```python
from build123d import *

# Parameters (mm, degrees)
ESQUISSE1_W             = 60
ESQUISSE1_H             = 42
BOSS_EXTRU_1_DEPTH      = 35.125
COQUE4_T                = -3
ESQUISSE7_W             = 54
ESQUISSE7_H             = 36
BOSS_EXTRU_2_DEPTH      = 10.125
ESQUISSE8_W             = 60
ESQUISSE8_H             = 35.125
ENL_V_MAT_EXTRU_1_DEPTH = 1
ESQUISSE9_W             = 10
ESQUISSE9_H             = 22
BOSS_EXTRU_3_DEPTH      = 1
ESQUISSE10_W            = 18
ESQUISSE10_H            = 10
ENL_V_MAT_EXTRU_2_DEPTH = 3
ESQUISSE13_W            = 42
ESQUISSE13_H            = 22
ENL_V_MAT_EXTRU_3_DEPTH = 10
ESQUISSE15_W            = 7.326333239
ESQUISSE15_H            = 18.950794871
ENL_V_MAT_EXTRU_4_DEPTH = 4
ESQUISSE16_W            = 5
ESQUISSE16_H            = 6
BOSS_EXTRU_4_DEPTH      = 3


with BuildPart() as part:
    # Esquisse1 → Boss.-Extru.1 (new body)
    with BuildSketch(Plane.XY):
        with Locations((30, 21)):
            Rectangle(ESQUISSE1_W, ESQUISSE1_H)
    extrude(amount=BOSS_EXTRU_1_DEPTH)

    # Coque4
    coque4_openings = [part.faces().sort_by_distance(p)[0] for p in [
        (30, 21, 35.125),
    ]]
    offset(amount=COQUE4_T, openings=coque4_openings, kind=Kind.INTERSECTION)

    # Esquisse7 → Boss.-Extru.2 (add)
    with BuildSketch(Plane.XY.offset(3)):
        with Locations((30, 21)):
            Rectangle(ESQUISSE7_W, ESQUISSE7_H)
    extrude(amount=BOSS_EXTRU_2_DEPTH)

    # Esquisse8 → Enlèv. mat.-Extru.1 (cut)
    with BuildSketch(Plane(origin=(0, 42, 0), x_dir=(1, 0, 0), z_dir=(0, 1, 0))):
        with Locations((30, -17.5625)):
            Rectangle(ESQUISSE8_W, ESQUISSE8_H)
    extrude(amount=-ENL_V_MAT_EXTRU_1_DEPTH, mode=Mode.SUBTRACT)

    # Esquisse9 → Boss.-Extru.3 (add)
    with BuildSketch(Plane(origin=(0, 41, 0), x_dir=(1, 0, 0), z_dir=(0, 1, 0))):
        with Locations((55, -24.125)):
            Rectangle(ESQUISSE9_W, ESQUISSE9_H)
    extrude(amount=-BOSS_EXTRU_3_DEPTH)

    # Esquisse10 → Enlèv. mat.-Extru.2 (cut)
    with BuildSketch(Plane.ZY):
        with Locations((22.395110195, 7.568318588)):
            Rectangle(ESQUISSE10_W, ESQUISSE10_H)
    extrude(amount=-ENL_V_MAT_EXTRU_2_DEPTH, mode=Mode.SUBTRACT)

    # Esquisse13 → Enlèv. mat.-Extru.3 (cut)
    with BuildSketch(Plane(origin=(0, 39, 0), x_dir=(-1, 0, 0), z_dir=(0, -1, 0))):
        with Locations((-24, -24.125)):
            Rectangle(ESQUISSE13_W, ESQUISSE13_H)
    extrude(amount=-ENL_V_MAT_EXTRU_3_DEPTH, mode=Mode.SUBTRACT)

    # Esquisse15 → Enlèv. mat.-Extru.4 (cut)
    with BuildSketch(Plane(origin=(0, 41, 0), x_dir=(1, 0, 0), z_dir=(0, 1, 0))):
        with Locations((48.66316662, -25.649602565)):
            Rectangle(ESQUISSE15_W, ESQUISSE15_H)
    extrude(amount=-ENL_V_MAT_EXTRU_4_DEPTH, mode=Mode.SUBTRACT)

    # Esquisse16 → Boss.-Extru.4 (add)
    with BuildSketch(Plane.XY.offset(13.125)):
        with Locations((5.5, 38)):
            Rectangle(ESQUISSE16_W, ESQUISSE16_H)
    extrude(amount=BOSS_EXTRU_4_DEPTH)


solid = part.part
```
For this review, take the finished solid that the model builds, in its own axes (mm). A direction names the side the tool comes from. Round coordinates to 2 decimals unless told otherwise and drop trailing zeros. Write each loop counter-clockwise with the first axis right and the second up, starting at its lowest first coordinate (ties: lowest second). Pieces come first, ordered by that corner, then holes. Notation, with made-up numbers: (-39.5, 15) - (-8.5, 15) arc R14 cw to (-8.5, 31) - close; hole circle Ø9 at (-3, -30.5). An arc over 180 degrees is marked (long way). Answer as a JSON object with one key per item and string values.
1. Tool access review of faces 5 (the face through (45, 40, 15)), 6 (the face through (1, 2.568, 22)), 7 (the face through (5, 35, 15)): name each direction out of +Z, -Z, +X, -X, +Y, -Y from which nothing blocks a thin tool from reaching the whole face with its end or side.
Response values:
{"face 5": "+Z, +Y", "face 6": "-X", "face 7": "+Z"}
2. We need section D-D on z = 32.5. Give the boundary of the cut face in (x, y).
Response values:
{"outline": "(0, 0) - (60, 0) - (60, 41) - (52.33, 41) - (52.33, 39) - (57, 39) - (57, 3) - (3, 3) - (3, 41) - (0, 41) - close"}
3. We need section A-A on z = 14.5. Give the boundary of the cut face in (x, y), then the cut area to 3 significant figures.
Response values:
{"outline": "(0, 0) - (60, 0) - (60, 41) - (45, 41) - (45, 39) - (57, 39) - (57, 3) - (3, 3) - (3, 2.57) - (0, 2.57) - close; (0, 12.57) - (3, 12.57) - (3, 35) - (8, 35) - (8, 41) - (0, 41) - close", "area": "432 mm2"}
4. We need section C-C on x = 48. Give the boundary of the cut face in (y, z) (3 decimals).
Response values:
{"outline": "(0, 0) - (41, 0) - (41, 16.174) - (39, 16.174) - (39, 13.125) - (3, 13.125) - (3, 35.125) - (0, 35.125) - close"}
5. To check wall thickness, follow line 1 along X through (y, z) = (14.5, 20.5); line 2 along X through (y, z) = (37.5, 14); line 3 along Z through (x, y) = (8.5, 10.5) (3 decimals). State the ranges of each line that lie inside material, in increasing order.
Response values:
{"line 1": "x = 0 to 3, 57 to 60", "line 2": "x = 0 to 8, 57 to 60", "line 3": "z = 0 to 13.125"}
6. Draft analysis for pull direction Z (two halves, no side actions). For faces 1 (the face through (32, 2, 35.125)), 2 (the face through (1, 7, 13.395)), 3 (the face through (1, 12.568, 22)), 4 (the face through (30, 21, 0)), state which applies: +Z half, -Z half, draft (parallel to the pull), parting line (faces both ways), or undercut.
Response values:
{"face 1": "+Z half", "face 2": "undercut", "face 3": "undercut", "face 4": "-Z half"}
7. We need section B-B on y = 22.5. Give the boundary of the cut face in (x, z) (3 decimals).
Response values:
{"outline": "(0, 0) - (60, 0) - (60, 35.125) - (57, 35.125) - (57, 13.125) - (3, 13.125) - (3, 35.125) - (0, 35.125) - close"}
8. For pin 1 Ø10 at (x, y) = (47, 31) entering from +Z (3 decimals); pin 2 Ø0.9 at (x, z) = (2, 23) entering from -Y; pin 3 Ø6.5 at (x, z) = (20.5, 19) entering from +Y; pin 4 Ø1.6 at (x, y) = (49, 40) entering from +Z, all flat-tipped, find the tip position at first contact; note any pin that passes through.
Response values:
{"pin 1": "stops at z = 13.125", "pin 2": "stops at y = 0", "pin 3": "stops at y = 3", "pin 4": "stops at z = 16.17"}
